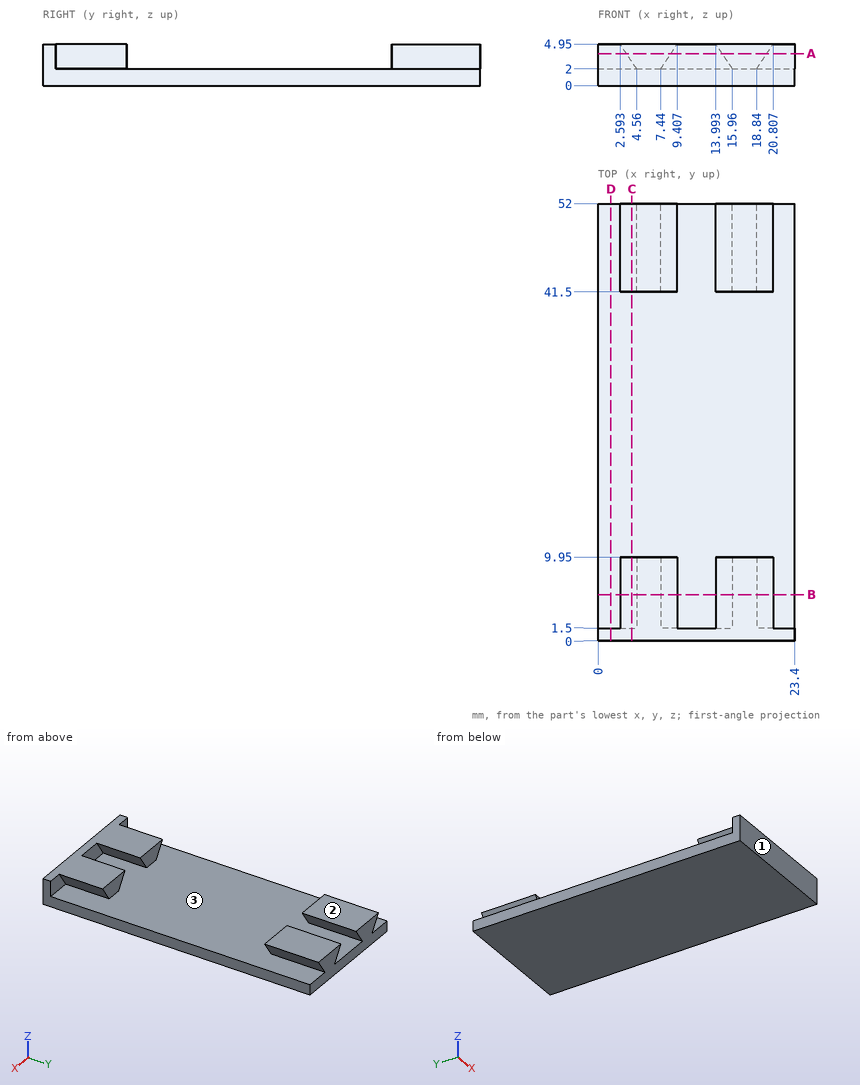
Job drawing, mm, ordinate dimensions from the low corner. One solid piece. Round coordinates to 2 decimals unless told otherwise and drop trailing zeros. Loops run counter-clockwise (first coordinate to the right, second up) from the corner with the lowest first, then second, coordinate; pieces in that order, holes last. Notation, with made-up numbers: (11, 73) -> (32, 73) arc R13 cw to (32, 86) -> close; hole circle Ø4 at (63, 75). An arc over 180 degrees is marked (long way). Use CSV: the item, a comma, the result in double quotes. Start each with the question number.
Q1. Saw through at D-D on x = 1.5. Give the cut face in (y, z).
Q2. Saw through at C-C on x = 4. Give the cut face in (y, z).
Q3. Flat gauge pins, fed straight in: pin 1 Ø2.5 at (x, z) = (1.5, 4) entering from +Y; pin 2 Ø2 at (x, y) = (9, 39.5) entering from +Z. Where does each tip first touch, or does it go through?
Q4. Drill centre lines: L1, parallel to Y at x = 16, z = 3.6; L2, parallel to Z at x = 22.25, y = 39.5; L3, parallel to Y at x = 12.5, z = 2.8. Where is each one in solid material? Low to high.
Q5. Saw through at B-B on y = 5.5. Give the cut face in (x, z).
Q6. Mould opens along Z. For the marked faces 1, 2 and 3 say: +Z half, -Z half, draft (parallel to the pull), parting line (faces both ways), or undercut.
Q7. Saw through at A-A on z = 3.8. Give the cut face in (x, y).
Solutions:
1,outline,"(0, 0) -> (52, 0) -> (52, 2) -> (1.5, 2) -> (1.5, 4.95) -> (0, 4.95) -> close"
2,outline,"(0, 0) -> (52, 0) -> (52, 2) -> (1.5, 2) -> (1.5, 2.84) -> (9.95, 2.84) -> (9.95, 4.95) -> (0, 4.95) -> close; (41.5, 2.84) -> (52, 2.84) -> (52, 4.95) -> (41.5, 4.95) -> close"
3,pin 1,"stops at y = 1.5"
3,pin 2,"stops at z = 2"
4,L1,"y = 0 to 9.95, 41.5 to 52"
4,L2,"z = 0 to 2"
4,L3,"y = 0 to 1.5"
5,outline,"(0, 0) -> (23.4, 0) -> (23.4, 2) -> (18.84, 2) -> (20.81, 4.95) -> (13.99, 4.95) -> (15.96, 2) -> (7.44, 2) -> (9.41, 4.95) -> (2.59, 4.95) -> (4.56, 2) -> (0, 2) -> close"
6,face 1,"draft"
6,face 2,"+Z half"
6,face 3,"undercut"
7,outline,"(0, 0) -> (23.4, 0) -> (23.4, 1.5) -> (20.04, 1.5) -> (20.04, 9.95) -> (14.76, 9.95) -> (14.76, 1.5) -> (8.64, 1.5) -> (8.64, 9.95) -> (3.36, 9.95) -> (3.36, 1.5) -> (0, 1.5) -> close; (3.36, 41.5) -> (8.64, 41.5) -> (8.64, 52) -> (3.36, 52) -> close; (14.76, 41.5) -> (20.04, 41.5) -> (20.04, 52) -> (14.76, 52) -> close"
